from build123d import *

# Parameters (mm, degrees)
F0_R     = 15.5
F1_DEPTH = 31
F2_R     = 15.5
F3_DEPTH = 16
F4_W     = 13.25
F4_H     = 13.25
F5_DEPTH = 16
F6_W     = 13.25
F6_H     = 1.5
F7_DEPTH = 0.25
F8_R     = 1


with BuildPart() as f1:
    # F0 (on Top) → F1 (new body)
    with BuildSketch(Plane.XY):
        Circle(F0_R)
        Polygon((-5.528129, 9.575), (5.528129, 9.575), (11.056258, 0), (5.528129, -9.575), (-5.528129, -9.575), (-11.056258, 0), align=None, mode=Mode.SUBTRACT)
    extrude(amount=F1_DEPTH)

    # F2 (on face) → F3 (join)
    with BuildSketch(Plane.XY.offset(31)):
        Circle(F2_R)
    extrude(amount=F3_DEPTH)

    # F4 (on face) → F5 (cut, through all)
    with BuildSketch(Plane.XY.offset(47)):
        Rectangle(F4_W, F4_H)
    extrude(amount=-F5_DEPTH, mode=Mode.SUBTRACT)

    # F6 (on face) → F7 (cut)
    with BuildSketch(Plane(origin=(6.625, 0, 0), x_dir=(0, -1, 0), z_dir=(-1, 0, 0))):
        with Locations((0, 40.95)):
            Rectangle(F6_W, F6_H)
    extrude(amount=-F7_DEPTH, mode=Mode.SUBTRACT)

    # F8
    f8_edges = [f1.edges().sort_by_distance(p)[0] for p in [
        (-15.5, 0, 0),
    ]]
    fillet(f8_edges, radius=F8_R)


solid = f1.part
Can you work these out from the model? Positions are in its coordinate system, mm. A direction names the side the tool comes from. Coordinates: 2 decimals unless noted, no trailing zeros. Write each loop counter-clockwise with the first axis right and the second up, starting at its lowest first coordinate (ties: lowest second). Pieces come first, ordered by that corner, then holes.
Q1. For P1, Ø1, axis at y = -7.5, z = 7, coming from the +X side; P2, Ø5, axis at y = 10.5, z = 8, coming from the +X side; P3, Ø8, axis at x = -5.5, y = -0.5, coming from the -Z side, each with a flat end and sliding along its axis, tell me the tip position at first contact or that it passes through.
Results found:
P1: stops at x = 13.83
P2: stops at x = 13.28
P3: stops at z = 31
Q2. Please list where these lines run through material, in increasing order: L1, parallel to Y at x = 5.5, z = 42 (3 decimals); L2, parallel to Y at x = 1, z = 29 (3 decimals).
Results found:
L1: y = -14.491 to -6.625, 6.625 to 14.491
L2: y = -15.468 to -9.575, 9.575 to 15.468
Q3. Imagine slicing it at B-B, the plane x = 0. List the corners of the cut face in (y, z) for me (3 decimals).
Results found:
outline: (-15.5, 1) arc R1 ccw to (-14.5, 0) - (-9.575, 0) - (-9.575, 31) - (-6.625, 31) - (-6.625, 47) - (-15.5, 47) - close; (6.625, 31) - (9.575, 31) - (9.575, 0) - (14.5, 0) arc R1 ccw to (15.5, 1) - (15.5, 47) - (6.625, 47) - close
Q4. If we mould it in two halves opening along X, with no side actions, what happens to faces 1 (the face through (-2.018, 15.368, 23.678)), 2 (the face through (9.5, 3.4, 0)), 3 (the face through (8.253, 4.855, 15.283))? For each: +X half, -X half, draft (parallel to the pull), parting line (faces both ways), or undercut.
Results found:
face 1: parting line
face 2: draft
face 3: undercut
Q5. Which directions (+Z, -Z, +X, -X, +Y, -Y) give clear straight access to the entire face, cutting with the end or side of a thin tool? Please do faces 4 (the face through (6.625, 0, 36)), 5 (the face through (0, 9.575, 15)), 6 (the face through (6.875, 0, 41)), 7 (the face through (0, -7, 47)).
Results found:
face 4: +Z, -Z
face 5: -Z
face 6: none
face 7: +Z, +X, -X, +Y, -Y
Q6. Imagine slicing it at A-A, the plane z = 19.5. List the corners of the cut face in (x, y) for me (3 decimals), plus the area to 3 significant figures.
Results found:
outline: circle Ø31 at (0, 0); hole (-11.056, 0) - (-5.528, -9.575) - (5.528, -9.575) - (11.056, 0) - (5.528, 9.575) - (-5.528, 9.575) - close
area: 437 mm2
